Autodesk Inventor part; units mm, degrees
ref_plane "YZ Plane" through (0, 0, 0) normal (1, 0, 0) x (0, 1, 0)
ref_plane "XZ Plane" through (0, 0, 0) normal (0, 1, 0) x (-1, 0, 0)
ref_plane "XY Plane" through (0, 0, 0) normal (0, 0, 1) x (1, 0, 0)
sketch "Sketch1" plane through (0, 0, 0) normal (1, 0, 0) x (0, 1, 0)
  line L0 (0, 0) -> (0, 44.45)
  arc A0 (0, 44.45) -> (-3.175, 40.1903) centre (-4.445, 44.45) ccw
  line L1 (-3.175, 40.1903) -> (-3.175, 0)
  line L2 (-3.175, 0) -> (0, 0)
  circle A1 centre (-1.5875, 0) radius 1.5875
  dimension "d0" = 3.175
  dimension "d1" = 44.45
  dimension "d2" = 4.445
extrude "Extrusion1" add sketch "Sketch1" along normal blind 6.35
sketch "Sketch2" plane through (6.35, 0, 0) normal (1, 0, 0) x (0, 0, -1)
  arc A0 (0, -3.175) -> (0, 0) centre (0, -1.5875) ccw
hole "Hole1" at (6.35, -1.5875, 0) direction (-1, 0, 0) diameter 1.5875 end through all
properties part number "Arm" material "Lead"
Geometry check sheet. Reference: the model listing, model coordinates, mm. Coordinates: 2 decimals unless noted, no trailing zeros. Loops run counter-clockwise (first coordinate to the right, second up) from the corner with the lowest first, then second, coordinate; pieces in that order, holes last. Notation, with made-up numbers: (39.5, 24.25) - (59.5, 24.25) arc R33 cw to (59.5, 60.25) - close; hole circle Ø3 at (11, -7.5). An arc over 180 degrees is marked (long way). One line per item, written item: value. Start each with the question number.
(1) Mould release check, pull along Z, two halves, no side actions. Record for faces 1 (the cylindrical face through (3.131, -2.257, -0.427)), 2 (the cylindrical face through (3.131, -1.553, -1.587)), 3 (the flat face through (0, -3, 30)): released by +Z, released by -Z, zero draft, split by the parting line, or undercut.
(2) Material ranges on line 1 (Y direction, x = 4, z = 0) (3 decimals); line 2 (Z direction, x = 5.5, y = -4.25); line 3 (Z direction, x = 5.25, y = -1.75), recorded low to high. Write a range as [from, to].
(3) Depth check by flat-ended pin: P1, Ø1.5, axis at x = 2.5, z = 33, coming from the -Y side (3 decimals); P2, Ø5, axis at y = -1.5, z = 6.5, coming from the -X side; P3, Ø2, axis at y = -6, z = 27.5, coming from the -X side. Enter the tip coordinate at first touch or a pass-through.
(4) Cross-section at B-B on z = 10. Enter the section's corners in (x, y) (3 decimals), plus the area to 3 significant figures.
Results below:
1. face 1: undercut
1. face 2: released by -Z
1. face 3: zero draft
2. line 1: y = [-3.175, -2.381], [-0.794, 0]
2. line 2: z = [40.01, 48.89]
2. line 3: z = [-1.58, -0.78], [0.78, 47.98]
3. P1: stops at y = -3.175
3. P2: stops at x = 0
3. P3: passes through
4. outline: (0, -3.175) - (6.35, -3.175) - (6.35, 0) - (0, 0) - close
4. area: 20.2 mm2
